from build123d import *

# Parameters (mm, degrees)
SKETCH1_W                                           = 120
SKETCH1_H                                           = 120
SKETCH1_R                                           = 47.5
BOSS_EXTRUDE1_DEPTH                                 = 18
SKETCH5_OUTSIDE_W                                   = 156.132
SKETCH5_OUTSIDE_H                                   = 156.132
SKETCH5_OUTSIDE_R                                   = 55
CUT_EXTRUDE1_DEPTH                                  = 5
SKETCH12_R                                          = 50
CUT_EXTRUDE2_DEPTH                                  = 12
CBORE_FOR_M6_HEX_SOCKET_HEAD_CAP_SCREW1_D           = 6.6
CBORE_FOR_M6_HEX_SOCKET_HEAD_CAP_SCREW1_CBORE_D     = 11
CBORE_FOR_M6_HEX_SOCKET_HEAD_CAP_SCREW1_CBORE_DEPTH = 7
CIRPATTERN1_COUNT                                   = 4
FILLET1_R                                           = 10
FILLET2_R                                           = 0.38
CHAMFER1_SIZE                                       = 0.7
M6_TAPPED_HOLE1_D                                   = 5
M8_TAPPED_HOLE1_D                                   = 6.8
M8_TAPPED_HOLE1_DEPTH                               = 32.99
M8_TAPPED_HOLE1_TIP                                 = 2.042926105
CHAMFER2_SIZE                                       = 1.524
CHAMFER2_SIZE2                                      = 0.87988181
SKETCH13_R                                          = 50.5
CUT_EXTRUDE3_DEPTH                                  = 1.524


with BuildPart() as part:
    # Sketch1 → Boss-Extrude1 (new body)
    with BuildSketch(Plane.XY):
        Rectangle(SKETCH1_W, SKETCH1_H)
        Circle(SKETCH1_R, mode=Mode.SUBTRACT)
    extrude(amount=-BOSS_EXTRUDE1_DEPTH)

    # Sketch5 outside → Cut-Extrude1 (cut)
    with BuildSketch(Plane(origin=(0, 0, -18), x_dir=(-1, 0, 0), z_dir=(0, 0, -1))):
        Rectangle(SKETCH5_OUTSIDE_W, SKETCH5_OUTSIDE_H)
        Circle(SKETCH5_OUTSIDE_R, mode=Mode.SUBTRACT)
    extrude(amount=-CUT_EXTRUDE1_DEPTH, mode=Mode.SUBTRACT)

    # Sketch12 → Cut-Extrude2 (cut)
    with BuildSketch(Plane.XY):
        Circle(SKETCH12_R)
    extrude(amount=-CUT_EXTRUDE2_DEPTH, mode=Mode.SUBTRACT)

    # CBORE for M6 Hex Socket Head Cap Screw1 (through all)
    with Locations(Plane.XY):
        with Locations((-52.827549631, 30.5), (-30.5, 52.827549631)):
            cbore_for_m6_hex_socket_head_cap_screw1 = CounterBoreHole(CBORE_FOR_M6_HEX_SOCKET_HEAD_CAP_SCREW1_D / 2, CBORE_FOR_M6_HEX_SOCKET_HEAD_CAP_SCREW1_CBORE_D / 2, CBORE_FOR_M6_HEX_SOCKET_HEAD_CAP_SCREW1_CBORE_DEPTH)

    # CirPattern1: CBORE for M6 Hex Socket Head Cap Screw1 ×4 about axis
    cirpattern1_axis = Axis((0, 0, 0), (0, 0, 1))
    for i in range(1, CIRPATTERN1_COUNT):
        add(cbore_for_m6_hex_socket_head_cap_screw1.rotate(cirpattern1_axis, i * 360 / CIRPATTERN1_COUNT), mode=Mode.SUBTRACT)

    # Fillet1
    fillet1_edges = [part.edges().sort_by_distance(p)[0] for p in [
        (-60, -60, -6.5),
        (60, -60, -6.5),
        (60, 60, -6.5),
        (-60, 60, -6.5),
    ]]
    fillet(fillet1_edges, radius=FILLET1_R)

    # Fillet2
    fillet2_edges = [part.edges().sort_by_distance(p)[0] for p in [
        (55, 0, -13),
    ]]
    fillet(fillet2_edges, radius=FILLET2_R)

    # Chamfer1
    chamfer1_edges = [part.edges().sort_by_distance(p)[0] for p in [
        (55, 0, -18),
    ]]
    chamfer(chamfer1_edges, length=CHAMFER1_SIZE)

    # M6 Tapped Hole1 (through all)
    with Locations(Plane.XY):
        with Locations((-43.133513652, -43.133513652), (-43.133513652, 43.133513652), (43.133513652, 43.133513652), (43.133513652, -43.133513652)):
            Hole(M6_TAPPED_HOLE1_D / 2)

    # M8 Tapped Hole1
    with Locations(Plane.XY):
        with Locations((-50, 50), (50, 50), (50, -50), (-50, -50)):
            Hole(M8_TAPPED_HOLE1_D / 2, depth=M8_TAPPED_HOLE1_DEPTH)
            with Locations((0, 0, -(M8_TAPPED_HOLE1_DEPTH + M8_TAPPED_HOLE1_TIP / 2))):  # 118° drill point
                Cone(0, M8_TAPPED_HOLE1_D / 2, M8_TAPPED_HOLE1_TIP, mode=Mode.SUBTRACT)

    # Chamfer2
    chamfer2_edges = [part.edges().sort_by_distance(p)[0] for p in [
        (-50, 0, 0),
    ]]
    chamfer2_side = [part.faces().sort_by_distance(p)[0] for p in [
        (-50, 0, -6),
    ]]
    chamfer(chamfer2_edges, length=CHAMFER2_SIZE, length2=CHAMFER2_SIZE2, reference=chamfer2_side[0])

    # Sketch13 → Cut-Extrude3 (cut)
    with BuildSketch(Plane.XY.offset(-12)):
        with Locations(Location((0, 0, 0), (0, 0, 180))):
            Circle(SKETCH13_R)
    extrude(amount=CUT_EXTRUDE3_DEPTH, mode=Mode.SUBTRACT)


solid = part.part
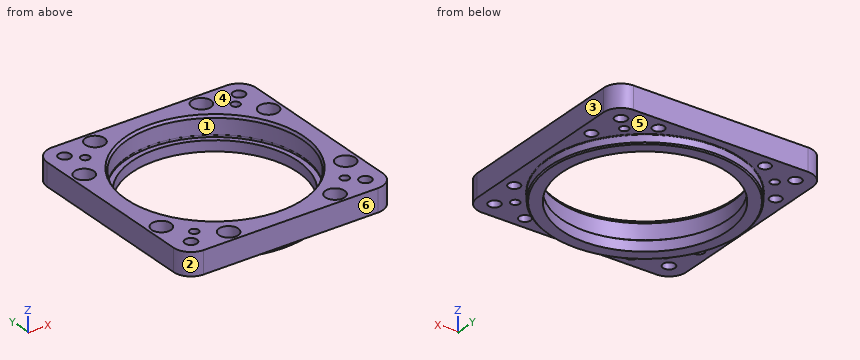
The model under review builds one solid part; all positions refer to its coordinate system, in mm. Face numbers are marked on the shaded views. A direction names the side the tool comes from. Round coordinates to 2 decimals unless told otherwise and drop trailing zeros. Order: outer loops, then holes, each group sorted by start corner. A loop starts at its lowest first (then second) coordinate and runs counter-clockwise, first axis right, second up. Notation, with made-up numbers: (80.25, 35.5) -> (131.25, 35.5) arc R30 cw to (131.25, 66.5) -> close; hole circle Ø8 at (23, -17). An arc over 180 degrees is marked (long way). Return JSON: item names as keys, results as strings.
1. Take a section at C-C (z = -4.5). State how many separate pieces and enclosed holes the cut face has, then the cut area to 3 significant figures.
Answer block:
{"separate pieces": "1", "enclosed holes": "17", "area": "5,480 mm²"}
2. For L1, parallel to X at y = -43, z = -4; L2, parallel to Y at x = -30.5, z = -8.55; L3, parallel to X at y = -1.5, z = -16.75, list the stretches that pass through material, from the lowest coordinate up. Write a range as [from, to].
Answer block:
{"L1": "x = [-60, -45.63], [-40.64, -25.51], [25.51, 40.64], [45.63, 60]", "L2": "y = [-60, -56.13], [-49.53, -39.62], [39.62, 49.53], [56.13, 60]", "L3": "x = [-54.98, -47.48], [47.48, 54.98]"}
3. The part is to be moulded in two halves that separate along X. For the marked faces 1, 2, 3 and 4, say which applies: +X half, -X half, draft (parallel to the pull), parting line (faces both ways), or undercut.
Answer block:
{"face 1": "undercut", "face 2": "-X half", "face 3": "+X half", "face 4": "draft"}
4. Take a section at A-A (x = 0). Write out the cut boundary in (y, z).
Answer block:
{"outline": "(-60, -13) -> (-55.38, -13) arc R0.38 cw to (-55, -13.38) -> (-55, -17.3) -> (-54.3, -18) -> (-47.5, -18) -> (-47.5, -12) -> (-50.5, -12) -> (-50.5, -10.48) -> (-50, -10.48) -> (-50, -1.52) -> (-50.88, 0) -> (-60, 0) -> close; (47.5, -18) -> (54.3, -18) -> (55, -17.3) -> (55, -13.38) arc R0.38 cw to (55.38, -13) -> (60, -13) -> (60, 0) -> (50.88, 0) -> (50, -1.52) -> (50, -10.48) -> (50.5, -10.48) -> (50.5, -12) -> (47.5, -12) -> close"}
5. Insertion check: P1, Ø12.5, axis at x = -52.83, y = 30.5, coming from the -Z side; P2, Ø2, axis at x = 31, z = -15.5, coming from the +Y side; P3, Ø7.5, axis at x = -52.83, y = -30.5, coming from the -Z side; P4, Ø6, axis at y = 2, z = -14.5, coming from the -X side. Each pin has a flat end and moves straight along its axis. Give the tip position at first contact, or say it passes through.
Answer block:
{"P1": "stops at z = -17.55", "P2": "stops at y = 46.1", "P3": "stops at z = -13", "P4": "stops at x = -60"}
6. For the marked faces 5 and 6, list the 3-axis set-ups (+Z, -Z, +X, -X, +Y, -Y) from which the entire face can be reached by the end or side of a thin tool; tool diameter is ignored.
Answer block:
{"face 5": "-Z", "face 6": "+Z, -Z, +X, -X, -Y"}
7. Take a section at D-D (z = -15.5). Write out the cut boundary in (x, y), then the cut area to 3 significant figures.
Answer block:
{"outline": "circle Ø110 at (0, 0); hole circle Ø95 at (0, 0)", "area": "2,420 mm²"}
